```python
from build123d import *

# Parameters (mm, degrees)
BOSS_EXTRUDE1_DEPTH         = 32.25
SKETCH2_R                   = 5.5
CUT_EXTRUDE1_DEPTH          = 6.8
LPATTERN1_COUNT             = 2
LPATTERN1_PITCH             = 50
LPATTERN1_COUNT_DIR2        = 2
LPATTERN1_PITCH_DIR2        = 50
MIRROR1_COPY_1_SKETCH_R     = 5.5
MIRROR1_COPY_1_DEPTH        = 6.8
MIRROR1_COPY_2_SKETCH_R     = 5.5
MIRROR1_COPY_2_DEPTH        = 6.8
MIRROR1_COPY_3_SKETCH_R     = 5.5
MIRROR1_COPY_3_DEPTH        = 6.8
SKETCH3_R                   = 3.3
CUT_EXTRUDE2_DEPTH          = 63.8
LPATTERN2_COUNT             = 2
LPATTERN2_PITCH             = 50
LPATTERN2_COUNT_DIR2        = 2
LPATTERN2_PITCH_DIR2        = 50
M10X1_25_TAPPED_HOLE1_D     = 8.8
M10X1_25_TAPPED_HOLE1_DEPTH = 10
M10X1_25_TAPPED_HOLE1_TIP   = 2.643786724
SKETCH6_R                   = 25
CUT_EXTRUDE4_DEPTH          = 60
SKETCH7_R                   = 0.6
SKETCH7_R_2                 = 1
CUT_EXTRUDE5_DEPTH          = 26
FILLET1_R                   = 5
FILLET2_R                   = 2
FILLET3_R                   = 1
SKETCH8_R                   = 17
BOSS_EXTRUDE2_DEPTH         = 6
SKETCH9_R                   = 25
BOSS_EXTRUDE3_DEPTH         = 1
FILLET5_R                   = 1
CUT_EXTRUDE6_DEPTH          = 87
CUT_EXTRUDE6_DEPTH_BACK     = 38
SKETCH10_R                  = 8


with BuildPart() as part:
    # Sketch1 → Boss-Extrude1 (new, symmetric)
    with BuildSketch(Plane(origin=(0, 0, 0), x_dir=(1, 0, 0), z_dir=(0, 1, 0))):
        Polygon((-32.5, 32.5), (-7.5, 32.5), (-6.5, 32.5), (-7.5, 27.5), (7.5, 27.5), (6.5, 32.5), (7.5, 32.5), (32.5, 32.5), (32.5, 7.5), (32.5, 6.5), (27.5, 7.5), (27.5, -7.5), (32.5, -6.5), (32.5, -7.5), (32.5, -32.5), (7.5, -32.5), (6.5, -32.5), (7.5, -27.5), (-7.5, -27.5), (-6.5, -32.5), (-7.5, -32.5), (-32.5, -32.5), (-32.5, -8), (-42.5, -8), (-42.5, 8), (-32.5, 8), align=None)
    extrude(amount=BOSS_EXTRUDE1_DEPTH, both=True)

    # Sketch2 → Cut-Extrude1 (cut)
    with BuildSketch(Plane(origin=(0, 32.25, 0), x_dir=(1, 0, 0), z_dir=(0, 1, 0))):
        with Locations(Location((-25, 25, 0), (0, 0, 270))):
            Circle(SKETCH2_R)
    cut_extrude1 = extrude(amount=-CUT_EXTRUDE1_DEPTH, mode=Mode.SUBTRACT)

    # LPattern1: Cut-Extrude1 2 × 2
    with Locations(*[(i * LPATTERN1_PITCH, 0, j * LPATTERN1_PITCH_DIR2) for i in range(LPATTERN1_COUNT) for j in range(LPATTERN1_COUNT_DIR2) if (i, j) != (0, 0)]):
        add(cut_extrude1, mode=Mode.SUBTRACT)

    # Mirror1: Cut-Extrude1 across plane
    add(cut_extrude1.mirror(Plane.ZX), mode=Mode.SUBTRACT)

    # Mirror1 copy 1 sketch → Mirror1 copy 1 (cut)
    with BuildSketch(Plane(origin=(0, -32.25, 50), x_dir=(1, 0, 0), z_dir=(0, -1, 0))):
        with Locations((-25, -25)):
            Circle(MIRROR1_COPY_1_SKETCH_R)
    extrude(amount=-MIRROR1_COPY_1_DEPTH, mode=Mode.SUBTRACT)

    # Mirror1 copy 2 sketch → Mirror1 copy 2 (cut)
    with BuildSketch(Plane(origin=(50, -32.25, 0), x_dir=(1, 0, 0), z_dir=(0, -1, 0))):
        with Locations((-25, -25)):
            Circle(MIRROR1_COPY_2_SKETCH_R)
    extrude(amount=-MIRROR1_COPY_2_DEPTH, mode=Mode.SUBTRACT)

    # Mirror1 copy 3 sketch → Mirror1 copy 3 (cut)
    with BuildSketch(Plane(origin=(50, -32.25, 50), x_dir=(1, 0, 0), z_dir=(0, -1, 0))):
        with Locations((-25, -25)):
            Circle(MIRROR1_COPY_3_SKETCH_R)
    extrude(amount=-MIRROR1_COPY_3_DEPTH, mode=Mode.SUBTRACT)

    # Sketch3 → Cut-Extrude2 (cut)
    with BuildSketch(Plane(origin=(0, 32.25, 0), x_dir=(1, 0, 0), z_dir=(0, 1, 0))):
        with Locations(Location((-25, 25, 0), (0, 0, 270))):
            Circle(SKETCH3_R)
    cut_extrude2 = extrude(amount=-CUT_EXTRUDE2_DEPTH, mode=Mode.SUBTRACT)

    # LPattern2: Cut-Extrude2 2 × 2
    with Locations(*[(i * LPATTERN2_PITCH, 0, j * LPATTERN2_PITCH_DIR2) for i in range(LPATTERN2_COUNT) for j in range(LPATTERN2_COUNT_DIR2) if (i, j) != (0, 0)]):
        add(cut_extrude2, mode=Mode.SUBTRACT)

    # M10x1.25 Tapped Hole1
    with Locations(Plane.ZY.offset(42.5)):
        with Locations((0, -21.25), (0, 14.25)):
            Hole(M10X1_25_TAPPED_HOLE1_D / 2, depth=M10X1_25_TAPPED_HOLE1_DEPTH)
            with Locations((0, 0, -(M10X1_25_TAPPED_HOLE1_DEPTH + M10X1_25_TAPPED_HOLE1_TIP / 2))):  # 118° drill point
                Cone(0, M10X1_25_TAPPED_HOLE1_D / 2, M10X1_25_TAPPED_HOLE1_TIP, mode=Mode.SUBTRACT)

    # Sketch6 → Cut-Extrude4 (cut)
    with BuildSketch(Plane(origin=(0, 32.25, 0), x_dir=(1, 0, 0), z_dir=(0, 1, 0))):
        with Locations(Location((0, 0, 0), (0, 0, 270))):
            Circle(SKETCH6_R)
    extrude(amount=-CUT_EXTRUDE4_DEPTH, mode=Mode.SUBTRACT)

    # Sketch7 → Cut-Extrude5 (cut)
    with BuildSketch(Plane.ZY.offset(42.5)):
        with Locations((-1.046113874, 15.75709023)):
            Circle(SKETCH7_R)
        with Locations((-1.046113874, -20.009379673)):
            Circle(SKETCH7_R_2)
    extrude(amount=-CUT_EXTRUDE5_DEPTH, mode=Mode.SUBTRACT)

    # Fillet1
    fillet1_edges = [part.edges().sort_by_distance(p)[0] for p in [
        (32.5, 0, 32.5),
        (-32.5, 0, 32.5),
        (-32.5, 0, -32.5),
        (32.5, 0, -32.5),
    ]]
    fillet(fillet1_edges, radius=FILLET1_R)

    # Fillet2
    fillet2_edges = [part.edges().sort_by_distance(p)[0] for p in [
        (-32.5, 0, 8),
        (-42.5, 0, 8),
        (-42.5, 0, -8),
        (-32.5, 0, -8),
    ]]
    fillet(fillet2_edges, radius=FILLET2_R)

    # Fillet3
    fillet3_edges = [part.edges().sort_by_distance(p)[0] for p in [
        (6.5, 0, 32.5),
        (-6.5, 0, 32.5),
        (-6.5, 0, -32.5),
        (6.5, 0, -32.5),
        (32.5, 0, -6.5),
        (32.5, 0, 6.5),
    ]]
    fillet(fillet3_edges, radius=FILLET3_R)



with BuildPart() as body_2:
    # Sketch8 → Boss-Extrude2 (new body)
    with BuildSketch(Plane(origin=(0, 32.25, 0), x_dir=(1, 0, 0), z_dir=(0, 1, 0))):
        with Locations(Location((0, 0, 0), (0, 0, 270))):
            Circle(SKETCH8_R)
    extrude(amount=BOSS_EXTRUDE2_DEPTH)


with BuildPart() as part_1:
    add(part.part)

    add(body_2.part)  # Boss-Extrude3 merges body 2
    # Sketch9 → Boss-Extrude3 (add)
    with BuildSketch(Plane(origin=(0, 32.25, 0), x_dir=(1, 0, 0), z_dir=(0, 1, 0))):
        with Locations(Location((0, 0, 0), (0, 0, 270))):
            Circle(SKETCH9_R)
    extrude(amount=-BOSS_EXTRUDE3_DEPTH)

    # Fillet5
    fillet5_edges = [part_1.edges().sort_by_distance(p)[0] for p in [
        (0, 38.25, -17),
    ]]
    fillet(fillet5_edges, radius=FILLET5_R)

    # Sketch10 → Cut-Extrude6 (cut, two sides: drawn at the far end of the back side and taken through both)
    with BuildSketch(Plane(origin=(0, 38.25, 0), x_dir=(1, 0, 0), z_dir=(0, 1, 0)).offset(-CUT_EXTRUDE6_DEPTH_BACK)):
        with Locations(Location((0, 0, 0), (0, 0, 270))):
            Circle(SKETCH10_R)
    extrude(amount=CUT_EXTRUDE6_DEPTH + CUT_EXTRUDE6_DEPTH_BACK, mode=Mode.SUBTRACT)


solid = part_1.part
```
Verification items for the finished model (mm, model axes). A direction names the side the tool comes from. Coordinates: 2 decimals unless noted, no trailing zeros. Write each loop counter-clockwise with the first axis right and the second up, starting at its lowest first coordinate (ties: lowest second). Pieces come first, ordered by that corner, then holes. Notation, with made-up numbers: M 61,-5 L 66,-5 A14 cw 66,16 Z; hole C 86,65 d5. An arc over 180 degrees is marked long. One line per item, written item: value.
Item 1: Mould release check, pull along X, two halves, no side actions. Record for faces 4 (the flat face through (7.114, 0.452, 29.429)), 5 (the cylindrical face through (-31.07, -0.45, 31)), 6 (the flat face through (-18, 0, 32.5)): pulls with the +X half, pulls with the -X half, needs draft (parallel to the pull), parting line crosses it, or undercut.
Check sheet entries:
face 4: undercut
face 5: pulls with the -X half
face 6: needs draft
Item 2: Section check D-D, the plane x = -18. Record the boundary of the cut face in (y, z), plus the area to 3 significant figures.
Check sheet entries:
outline: M -32.25,-32.5 L 32.25,-32.5 L 32.25,32.5 L -32.25,32.5 Z; hole M -27.75,-17.35 L 31.25,-17.35 L 31.25,17.35 L -27.75,17.35 Z
area: 2,150 mm^2
Item 3: Section check A-A, the plane z = 26.5. Record the boundary of the cut face in (x, y), plus the area to 3 significant figures.
Check sheet entries:
outline: M -32.5,-32.25 L -30.29,-32.25 L -30.29,-25.45 L -27.94,-25.45 L -27.94,25.45 L -30.29,25.45 L -30.29,32.25 L -32.5,32.25 Z; M -22.06,-25.45 L -19.71,-25.45 L -19.71,-32.25 L 19.71,-32.25 L 19.71,-25.45 L 22.06,-25.45 L 22.06,25.45 L 19.71,25.45 L 19.71,32.25 L -19.71,32.25 L -19.71,25.45 L -22.06,25.45 Z; M 27.94,-25.45 L 30.29,-25.45 L 30.29,-32.25 L 32.5,-32.25 L 32.5,32.25 L 30.29,32.25 L 30.29,25.45 L 27.94,25.45 Z
area: 3,310 mm^2
Item 4: Scan lines: line 1 along Z through (x, y) = (25, -28.25); line 2 along X through (y, z) = (22, -22); line 3 along Z through (x, y) = (23, 29). Record each from-to range of solid material in increasing order.
Check sheet entries:
line 1: z = -32.5 to -30.5, -19.5 to 19.5, 30.5 to 32.5
line 2: x = -32.5 to -26.37, -23.63 to -11.87, 11.87 to 23.63, 26.37 to 32.5
line 3: z = -32.5 to -30.12, -19.88 to -9.8, 9.8 to 19.88, 30.12 to 32.5
Item 5: Access from +Z, -Z, +X, -X, +Y, -Y to the whole of each face (thin tool, end or side, straight path). Record for faces 1 (the flat face through (25, -25.45, -29)), 2 (the flat face through (-38, 0, -8)), 3 (the flat face through (6, 31.25, -6)).
Check sheet entries:
face 1: -Y
face 2: -Z, -X, +Y, -Y
face 3: none
Item 6: Section check C-C, the plane y = 7. State how many separate pieces and enclosed holes the cut face has, plus the area to 3 significant figures.
Check sheet entries:
separate pieces: 1
enclosed holes: 5
area: 2,050 mm^2
Item 7: Section check B-B, the plane x = 0. Record the boundary of the cut face in (y, z).
Check sheet entries:
outline: M -32.25,-27.5 L 32.25,-27.5 L 32.25,-17 L 37.25,-17 A1 ccw 38.25,-16 L 38.25,-8 L 31.25,-8 L 31.25,-25 L -27.75,-25 L -27.75,25 L 31.25,25 L 31.25,8 L 38.25,8 L 38.25,16 A1 ccw 37.25,17 L 32.25,17 L 32.25,27.5 L -32.25,27.5 Z
Item 8: Gauge pin test, flat ends, axial feed: pin 1 Ø1.5 at (x, y) = (-7.5, 7.5) entering from +Z; pin 2 Ø1 at (y, z) = (28, -15) entering from -X; pin 3 Ø1.5 at (x, z) = (-11, -19.5) entering from +Y; pin 4 Ø6.5 at (x, z) = (-25, -25) entering from -Y. Record the tip position at first contact, or that the pin passes through.
Check sheet entries:
pin 1: stops at z = 32.5
pin 2: stops at x = -32.5
pin 3: stops at y = 32.25
pin 4: passes through
